```python
from build123d import *

# Parameters (mm, degrees)
RESSALTO_EXTRUS_O1_DEPTH      = 3
ESBO_O1_3_W                   = 16.6
ESBO_O1_3_H                   = 23
ESBO_O1_3_R                   = 1.5
ESBO_O1_3_R_2                 = 0.5
RESSALTO_EXTRUS_O2_DEPTH      = 6
CORTE_EXTRUS_O1_DEPTH         = 3
CORTE_EXTRUS_O2_DEPTH         = 3
CHANFRO1_SIZE                 = 6
FURO_ROSCADO_DE_M3X0_51_D     = 2.5
FURO_ROSCADO_DE_M3X0_51_DEPTH = 8.5
FURO_ROSCADO_DE_M3X0_51_TIP   = 0.751075774
FURO_ROSCADO_DE_M3X0_52_D     = 2.5
FURO_ROSCADO_DE_M3X0_53_D     = 2.5
FURO_ROSCADO_DE_M3X0_53_DEPTH = 3
FURO_ROSCADO_DE_M3X0_53_TIP   = 0.751075774
ESBO_O17_R                    = 2.45
RESSALTO_EXTRUS_O3_DEPTH      = 3.5
CHANFRO2_SIZE                 = 0.5
FURO_ROSCADO_DE_M4X0_73_D     = 3.3
FURO_ROSCADO_DE_M4X0_73_DEPTH = 11.5
FURO_ROSCADO_DE_M4X0_73_TIP   = 0.991420021


with BuildPart() as part:
    # Esboço1 → Ressalto-extrusão1 (new body)
    with BuildSketch(Plane.XY):
        with BuildLine():
            Line((0, -2), (0, 0))
            Line((0, 0), (0, 16))
            ThreePointArc((0, 16), (-1.757359313, 11.757359313), (-6, 10))
            ThreePointArc((-6, 10), (-12, 4), (-6, -2))
            Line((-6, -2), (0, -2))
        make_face()
    extrude(amount=RESSALTO_EXTRUS_O1_DEPTH)

    # Esboço1<3> → Ressalto-extrusão2 (add)
    with BuildSketch(Plane.XY):
        with Locations((8.3, 11.5)):
            Rectangle(ESBO_O1_3_W, ESBO_O1_3_H)
        with Locations((11.6, 17.6)):
            Circle(ESBO_O1_3_R, mode=Mode.SUBTRACT)
        with Locations((4.68, 17.61)):
            Circle(ESBO_O1_3_R_2, mode=Mode.SUBTRACT)
    extrude(amount=RESSALTO_EXTRUS_O2_DEPTH)


with BuildPart() as body_2:
    # Espelhar1: mirrored copy
    add(part.part.mirror(Plane.XY.offset(6)))

    # Esboço4 → Corte-extrusão1 (cut)
    with BuildSketch(Plane(origin=(0, 0, 6), x_dir=(-1, 0, 0), z_dir=(0, 0, -1))):
        Polygon((0, 3.633024279), (-2.37796561, 23), (0, 23), align=None)
    extrude(amount=-CORTE_EXTRUS_O1_DEPTH, mode=Mode.SUBTRACT)

    # Esboço5 → Corte-extrusão2 (cut)
    with BuildSketch(Plane(origin=(0, 0, 9), x_dir=(-1, 0, 0), z_dir=(0, 0, -1))):
        with BuildLine():
            Line((-0.68649297, 9.224060849), (5.26878394, 9.95527691))
            ThreePointArc((5.26878394, 9.95527691), (5.633708763, 9.988808791), (6, 10))
            ThreePointArc((6, 10), (1.757359313, 11.757359313), (0, 16))
            Line((0, 16), (0, 23))
            Line((0, 23), (-2.37796561, 23))
            Line((-2.37796561, 23), (-0.68649297, 9.224060849))
        make_face()
    extrude(amount=-CORTE_EXTRUS_O2_DEPTH, mode=Mode.SUBTRACT)

    # Chanfro1
    # the kernel refuses this chamfer: 6 mm, written as the material it adds along each edge
    with BuildSketch(Plane(origin=(0.68649297, 9.224060849, 9), x_dir=(-0.9955217911555101, 0.09453234015153285, 0), z_dir=(0, 0, 1))) as chanfro1_piece_1:
        Polygon((CHANFRO1_SIZE * 0.999621916911, -CHANFRO1_SIZE * 0.0274958766106), (-CHANFRO1_SIZE * 0.0274958766106, -CHANFRO1_SIZE * 0.999621916911), (0, 0), align=None)
    extrude(amount=3)

    # Furo roscado de M3x0.51
    with Locations(Plane.XZ):
        with Locations((4, 9), (12.6, 9)):
            Hole(FURO_ROSCADO_DE_M3X0_51_D / 2, depth=FURO_ROSCADO_DE_M3X0_51_DEPTH)
            with Locations((0, 0, -(FURO_ROSCADO_DE_M3X0_51_DEPTH + FURO_ROSCADO_DE_M3X0_51_TIP / 2))):  # 118° drill point
                Cone(0, FURO_ROSCADO_DE_M3X0_51_D / 2, FURO_ROSCADO_DE_M3X0_51_TIP, mode=Mode.SUBTRACT)

    # Furo roscado de M3x0.52 (through all)
    with Locations(Plane(origin=(0, 0, 6), x_dir=(-1, 0, 0), z_dir=(0, 0, -1))):
        with Locations((-4.68, 17.61)):
            Hole(FURO_ROSCADO_DE_M3X0_52_D / 2)

    # Furo roscado de M3x0.53
    with Locations(Plane(origin=(0, 23, 0), x_dir=(-1, 0, 0), z_dir=(0, 1, 0))):
        with Locations((-8.1, 9)):
            Hole(FURO_ROSCADO_DE_M3X0_53_D / 2, depth=FURO_ROSCADO_DE_M3X0_53_DEPTH)
            with Locations((0, 0, -(FURO_ROSCADO_DE_M3X0_53_DEPTH + FURO_ROSCADO_DE_M3X0_53_TIP / 2))):  # 118° drill point
                Cone(0, FURO_ROSCADO_DE_M3X0_53_D / 2, FURO_ROSCADO_DE_M3X0_53_TIP, mode=Mode.SUBTRACT)

    # Esboço17 → Ressalto-extrusão3 (add)
    with BuildSketch(Plane(origin=(0, 0, 9), x_dir=(-1, 0, 0), z_dir=(0, 0, -1))):
        with Locations((6, 4)):
            Circle(ESBO_O17_R)
    extrude(amount=RESSALTO_EXTRUS_O3_DEPTH)

    # Chanfro2
    chanfro2_edges = [body_2.edges().sort_by_distance(p)[0] for p in [
        (-3.55, 4, 5.5),
    ]]
    chamfer(chanfro2_edges, length=CHANFRO2_SIZE)

    # Furo roscado de M4x0.73
    with Locations(Plane(origin=(0, 0, 6), x_dir=(-1, 0, 0), z_dir=(0, 0, -1))):
        with Locations((-11.6, 17.6)):
            Hole(FURO_ROSCADO_DE_M4X0_73_D / 2, depth=FURO_ROSCADO_DE_M4X0_73_DEPTH)
            with Locations((0, 0, -(FURO_ROSCADO_DE_M4X0_73_DEPTH + FURO_ROSCADO_DE_M4X0_73_TIP / 2))):  # 118° drill point
                Cone(0, FURO_ROSCADO_DE_M4X0_73_D / 2, FURO_ROSCADO_DE_M4X0_73_TIP, mode=Mode.SUBTRACT)


solid = body_2.part
```
Work out the finished part from the listing and answer in its coordinate system (mm). A direction names the side the tool comes from. Round coordinates to 2 decimals unless told otherwise and drop trailing zeros. Write each loop counter-clockwise with the first axis right and the second up, starting at its lowest first coordinate (ties: lowest second). Pieces come first, ordered by that corner, then holes. Notation, with made-up numbers: (22, 55.25) - (39, 55.25) arc R16 ccw to (39, 83.25) - close; hole circle Ø6 at (-16, -12.5). An arc over 180 degrees is marked (long way). Return JSON: item names as keys, results as strings. Group by question number.
Q1. Find the intervals of material crossed by L1, parallel to Z at x = 12.6, y = 4; L2, parallel to Y at x = 4.68, z = 10.75; L3, parallel to Z at x = 7.5, y = 16.5, in increasing order.
Q2. The part is cut by section C-C on y = 11.25. Write down the section's boundary in (x, z), then the cut area to 3 significant figures.
Q3. The part is cut by section A-A on z = 6.5. Write down the section's boundary in (x, y).
Q4. The part is cut by section B-B on y = 14.5. Write down the section's boundary in (x, z).
Q5. For faces 1 (the cylindrical face through (-8.337, 4.736, 7.521)), 2 (the flat face through (8, 12, 6)), 3 (the cylindrical face through (8.772, 21.479, 10.054)), 4 (the flat face through (0, -1, 11)), 5 (the cylindrical face through (12.76, 4.31, 10.24)), determine the directions among +Z, -Z, +X, -X, +Y, -Y from which every point of the face is accessible in a straight line to the end or side of a thin tool.
Q6. Each of these flat-tipped pins is pushed along its axis until it touches: pin 1 Ø3 at (x, z) = (6.5, 10) entering from -Y; pin 2 Ø1 at (x, y) = (7, 5) entering from -Z; pin 3 Ø3 at (y, z) = (13, 8.5) entering from -X. Where does it stop, or does it pass through?
Q7. The mould has two halves that part along X. Classify faces 6 (the flat face through (16.6, 11, 9)), 7 (the flat face through (-3, 5, 9)), 8 (the flat face through (-6, 4, 5.5)), 9 (the flat face through (0, 2, 8)): released by +X, released by -X, zero draft, split by the parting line, or undercut.
Solved:
{
 "1": {"L1": "6 to 7.75, 10.25 to 12", "L2": "0 to 16.36, 18.86 to 23", "L3": "6 to 12"},
 "2": {"outline": "(-3.61, 9) - (0.94, 9) - (0.94, 6) - (16.6, 6) - (16.6, 12) - (-3.61, 12) - close", "area": "108 mm²"},
 "3": {"outline": "circle Ø4.9 at (-6, 4); (0, 0) - (16.6, 0) - (16.6, 23) - (2.38, 23) - (0, 3.63) - close; hole circle Ø2.5 at (4.68, 17.61); hole circle Ø3.3 at (11.6, 17.6)"},
 "4": {"outline": "(0.55, 9) - (1.33, 9) - (1.33, 6) - (16.6, 6) - (16.6, 12) - (0.55, 12) - close"},
 "5": {"face 1": "-Z", "face 2": "-Z, +X, +Y, -Y", "face 3": "+Y", "face 4": "+Z, -Z, +X, -Y", "face 5": "-Y"},
 "6": {"pin 1": "y = 0", "pin 2": "z = 6", "pin 3": "x = -3.18"},
 "7": {"face 6": "released by +X", "face 7": "undercut", "face 8": "zero draft", "face 9": "undercut"}
}
